The drawing under review shows one solid part. Ordinate dimensions are in mm from its lowest x, y, z. A direction names the side the tool comes from. Coordinates: 2 decimals unless noted, no trailing zeros. Loops run counter-clockwise (first coordinate to the right, second up) from the corner with the lowest first, then second, coordinate; pieces in that order, holes last. Notation, with made-up numbers: (51.25, -38) - (102.25, -38) arc R16 cw to (102.25, -33) - close; hole circle Ø3 at (3, -11). An arc over 180 degrees is marked (long way). Answer as a JSON object with one key per item and string values. Group by question number.
Item 1: We need section B-B (z = 6.5). Give the boundary of the cut face in (x, y).
Item 2: We need section A-A (x = 4). Give the boundary of the cut face in (y, z) (1 decimal).
Item 3: We need section D-D (y = 9.25). Give the boundary of the cut face in (x, z), then the cut area to 3 significant figures.
Item 4: We need section C-C (z = 3.5). Give the boundary of the cut face in (x, y).
Item 5: To check wall thickness, follow line 1 (X direction, y = 3.5, z = 10.5); line 2 (Z direction, x = 16.5, y = 5); line 3 (Y direction, x = 2.25, z = 5.25). State the ranges of each line that lie inside material, in increasing order.
Item 6: Tool access review of the marked faces 1, 2, 3 and 4: name each direction out of +Z, -Z, +X, -X, +Y, -Y from which nothing blocks a thin tool from reaching the whole face with its end or side.
Item 7: Clearance check with flat-ended pins moving along their axes: pin 1 (6 mm diameter, centred on x = 15.5, y = 6, fed in from +Z); pin 2 (2 mm diameter, centred on x = 12, z = 9.5, fed in from -Y); pin 3 (3 mm diameter, centred on x = 16.5, y = 3, fed in from +Z); pin 4 (3 mm diameter, centred on x = 16, y = 6, fed in from -Z). State where each tip first meets the part, or that it passes through.
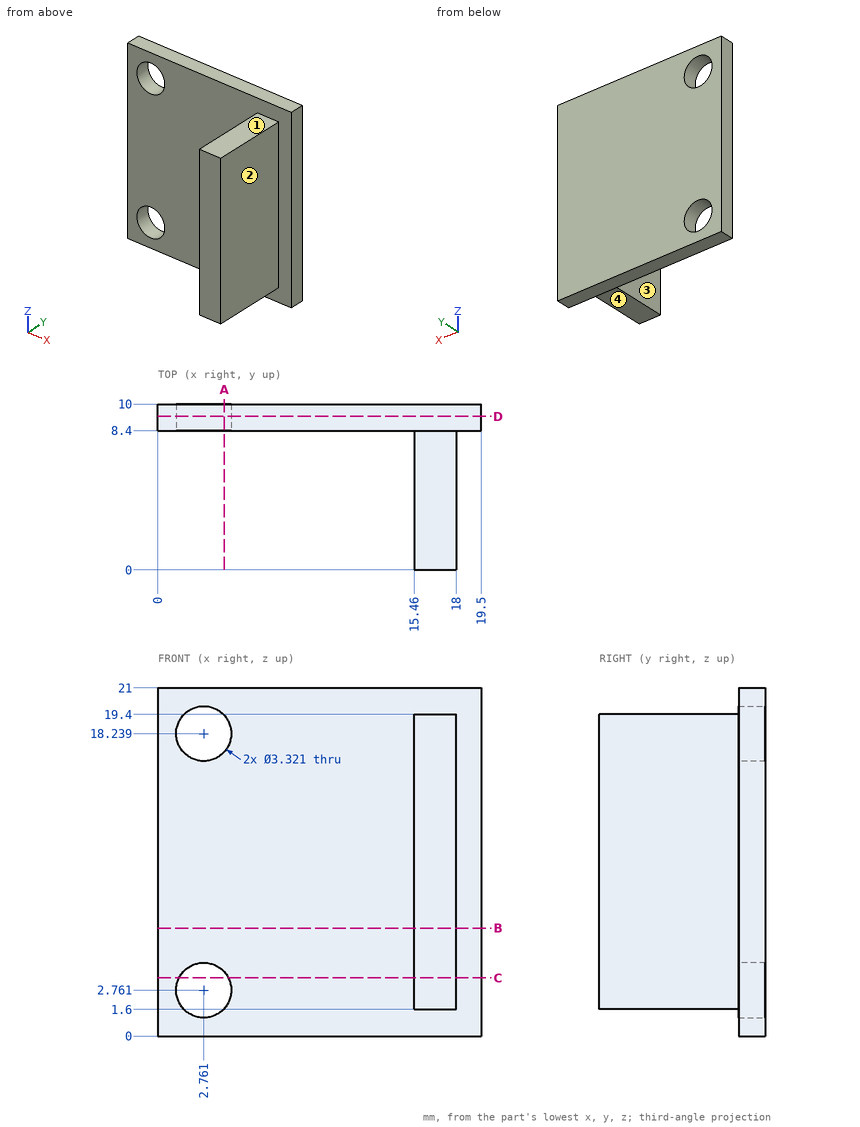
Check sheet entries:
{
 "1": {"outline": "(0, 8.4) - (15.46, 8.4) - (15.46, 0) - (18, 0) - (18, 8.4) - (19.5, 8.4) - (19.5, 10) - (0, 10) - close"},
 "2": {"outline": "(8.4, 0) - (10, 0) - (10, 1.7) - (8.4, 1.7) - close; (8.4, 3.9) - (10, 3.9) - (10, 17.1) - (8.4, 17.1) - close; (8.4, 19.3) - (10, 19.3) - (10, 21) - (8.4, 21) - close"},
 "3": {"outline": "(0, 0) - (19.5, 0) - (19.5, 21) - (0, 21) - close; hole circle Ø3.32 at (2.76, 2.76); hole circle Ø3.32 at (2.76, 18.24)", "area": "392 mm2"},
 "4": {"outline": "(0, 8.4) - (1.27, 8.4) - (1.27, 10) - (0, 10) - close; (4.25, 8.4) - (15.46, 8.4) - (15.46, 0) - (18, 0) - (18, 8.4) - (19.5, 8.4) - (19.5, 10) - (4.25, 10) - close"},
 "5": {"line 1": "x = 15.46 to 18", "line 2": "z = 1.6 to 19.4", "line 3": "y = 8.4 to 10"},
 "6": {"face 1": "+Z, +X, -X, -Y", "face 2": "+Z, -Z, +X, -Y", "face 3": "+Z, -Z, -X, -Y", "face 4": "-Z, +X, -X, -Y"},
 "7": {"pin 1": "stops at z = 21", "pin 2": "stops at y = 8.4", "pin 3": "stops at z = 19.4", "pin 4": "stops at z = 1.6"}
}
